```python
from build123d import *

# Parameters (mm, degrees)
BOSS_EXTRUDE1_DEPTH = 13.5
CHAMFER1_SIZE       = 0.75
CHAMFER2_SIZE       = 0.75
SCALE1_SCALE        = 0.9


with BuildPart() as part:
    # Sketch1 → Boss-Extrude1 (new body)
    # profile 1 of 3: a face of its own
    with BuildSketch(Plane.XY):
        with BuildLine():
            Line((-6.750000000000002, 15.249999999999998), (-6.750000000000003, 20.93889920697836))
            ThreePointArc((-6.750000000000044, 20.93889920697837), (-22, -1.685e-14), (-6.750000000000026, -20.938899206978377))
            Line((-6.749999999999997, -20.938899206978377), (-6.749999999999998, -15.25000000517543))
            Line((-6.749999999999998, -15.25000000517543), (-6.750000000000002, 15.249999999999998))
        make_face()
    # profile 2 of 3: a face of its own
    with BuildSketch(Plane.XY):
        with BuildLine():
            ThreePointArc((22, 0), (17.78341924377873, 12.95183384698863), (6.749999999999977, 20.93889920697839))
            Line((6.749999999999997, 20.938899206978398), (6.749999999999998, 15.25))
            Line((6.749999999999998, 15.25), (6.750000000000002, -15.25))
            Line((6.750000000000002, -15.25), (6.750000000000003, -20.93889920697839))
            ThreePointArc((6.749999999999982, -20.938899206978387), (17.78341924377873, -12.95183384698863), (22, -5.39e-15))
        make_face()
    # profile 3 of 3: a face of its own
    with BuildSketch(Plane.XY):
        with BuildLine():
            ThreePointArc((6.749999999999999, 15.249999999999998), (-1.24e-15, 8.5), (-6.749999999999999, 15.25))
            Line((-6.750000000000002, 15.249999999999998), (-6.749999999999998, -15.25000000517543))
            ThreePointArc((-6.75, -15.250000005175428), (-2.58771413e-09, -8.5), (6.75, -15.25))
            Line((6.750000000000002, -15.25), (6.749999999999998, 15.25))
        make_face()
        with BuildLine():
            Line((-0.8750000000000007, 3.7749172176354118), (-0.8750000000000008, 4.875))
            Line((-0.8750000000000008, 4.875), (0.8749999999999992, 4.875))
            Line((0.8749999999999992, 4.875), (0.8749999999999993, 3.774917217635379))
            ThreePointArc((0.8749999999999902, 3.774917217635377), (3.033665274877896, 2.4109126902482427), (3.875, 0))
            ThreePointArc((3.875, -9.5e-16), (3.033665274877896, -2.4109126902482427), (0.8749999999999918, -3.7749172176353767))
            Line((0.8750000000000004, -3.7749172176353767), (0.8750000000000006, -4.875))
            Line((0.8750000000000006, -4.875), (-0.8749999999999994, -4.875))
            Line((-0.8749999999999994, -4.875), (-0.8749999999999996, -3.774917217635412))
            ThreePointArc((-0.8749999999999161, -3.7749172176353945), (-3.875, 4.7e-16), (-0.8749999999999168, 3.774917217635394))
        make_face(mode=Mode.SUBTRACT)
    extrude(amount=BOSS_EXTRUDE1_DEPTH)

    # Chamfer1
    chamfer1_edges = [part.edges().sort_by_distance(p)[0] for p in [
        (-0.8749999999999996, -4.324958608817706, 0),
        (5.6e-16, -4.875, 0),
        (0.8750000000000004, -4.324958608817688, 0),
        (3.875, 1.22e-15, 0),
        (0.8749999999999993, 4.324958608817689, 0),
        (-7.8e-16, 4.875, 0),
        (-0.8750000000000007, 4.324958608817706, 0),
        (-3.8749999999999996, -3.3e-16, 0),
    ]]
    chamfer(chamfer1_edges, length=CHAMFER1_SIZE)

    # Chamfer2
    chamfer2_edges = [part.edges().sort_by_distance(p)[0] for p in [
        (-3.8749999999999996, -3.3e-16, 13.5),
        (-0.8750000000000007, 4.324958608817706, 13.5),
        (-7.8e-16, 4.875, 13.5),
        (0.8749999999999993, 4.324958608817689, 13.5),
        (3.875, -2.2e-16, 13.5),
        (0.8750000000000004, -4.324958608817688, 13.5),
        (5.6e-16, -4.875, 13.5),
        (-0.8749999999999996, -4.324958608817706, 13.5),
    ]]
    chamfer(chamfer2_edges, length=CHAMFER2_SIZE)


with BuildPart() as part_1:
    # Scale1: scaled about (0, 0, 6.75)
    add(part.part.scale(SCALE1_SCALE).moved(Location((0, 0, 0.6749999999999998))))


solid = part_1.part
```
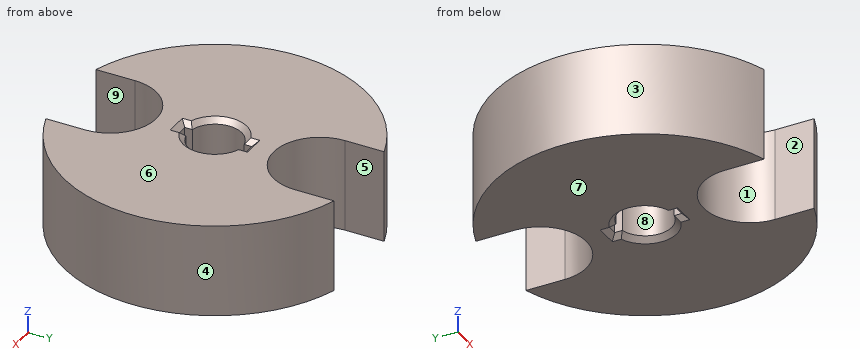
Design review of the part built by this model. Coordinates are the model's own, in mm. Face numbers are marked on the shaded views. A direction names the side the tool comes from. Give positions to 0.01 mm unless a question says otherwise; leave off trailing zeros. Write each loop counter-clockwise with the first axis right and the second up, starting at its lowest first coordinate (ties: lowest second). Pieces come first, ordered by that corner, then holes.
(1) Add section D-D (x = 14). Give the boundary of the cut face in (y, z) (3 decimals), and give its area (3 significant figures).
Checked values:
outline: (-14.001, 0.675) - (14.001, 0.675) - (14.001, 12.825) - (-14.001, 12.825) - close
area: 340 mm2
(2) Mouldability with a two-part tool opening along X and no side actions: class the marked faces 1, 2, 3 and 4 as +X half, -X half, draft (parallel to the pull), parting line (faces both ways), or undercut.
Checked values:
face 1: undercut
face 2: undercut
face 3: -X half
face 4: +X half
(3) Tool access review of the marked faces 5, 6, 7, 8 and 9: name each direction out of +Z, -Z, +X, -X, +Y, -Y from which nothing blocks a thin tool from reaching the whole face with its end or side.
Checked values:
face 5: +Z, -Z, +Y
face 6: +Z, +X, -X, +Y, -Y
face 7: -Z, +X, -X, +Y, -Y
face 8: +Z, -Z
face 9: +Z, -Z, -Y
(4) Add section C-C (y = 12). Give the boundary of the cut face in (x, z) (3 decimals).
Checked values:
outline: (-15.749, 0.675) - (-5.825, 0.675) - (-5.825, 12.825) - (-15.749, 12.825) - close; (5.825, 0.675) - (15.749, 0.675) - (15.749, 12.825) - (5.825, 12.825) - close
(5) Wall thickness on line 1 along X through (y, z) = (17, 8) (3 decimals); line 2 along X through (y, z) = (-13.5, 3.5); line 3 along Y through (x, z) = (-10.5, 9.5): over which ranges is each line inside the solid? List them lowest first.
Checked values:
line 1: x = -10.151 to -6.075, 6.075 to 10.151
line 2: x = -14.48 to -6.07, 6.07 to 14.48
line 3: y = -16.79 to 16.79
(6) Clearance check with flat-ended pins moving along their axes: pin 1 Ø1.1 at (y, z) = (4, 6) entering from -X; pin 2 Ø0.5 at (x, z) = (0, 9.5) entering from -Y; pin 3 Ø1.7 at (x, z) = (0, 9) entering from +Y. State where each tip first meets the part, or that it passes through.
Checked values:
pin 1: stops at x = -19.5
pin 2: stops at y = -7.66
pin 3: stops at y = 7.71
